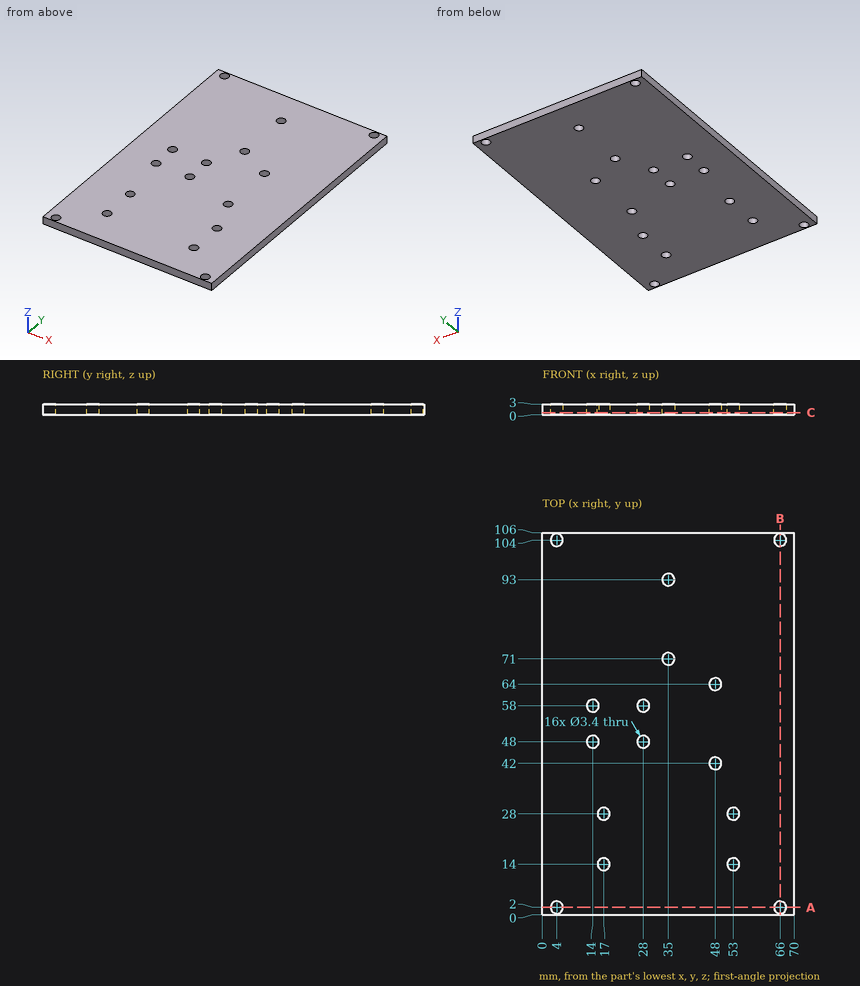
Part print with two shaded views. Sizes in mm from the minimum x, y, z corner. Coordinates: 2 decimals unless noted, no trailing zeros. Write each loop counter-clockwise with the first axis right and the second up, starting at its lowest first coordinate (ties: lowest second). Pieces come first, ordered by that corner, then holes. Notation, with made-up numbers: (-17, 14.25) - (15, 14.25) arc R18 ccw to (15, 48.25) - close; hole circle Ø8 at (16.25, -29.5). An arc over 180 degrees is marked (long way). Put each result on its own line as item: value.
1. Probe line 1 along Y through (x, z) = (66, 1.95); line 2 along Y through (x, z) = (35, 1.7); line 3 along X through (y, z) = (65, 1.7). List the from-to ranges inside material, lowest first. Write a range as [from, to].
Final values:
line 1: y = [0, 0.3], [3.7, 102.3], [105.7, 106]
line 2: y = [0, 69.3], [72.7, 91.3], [94.7, 106]
line 3: x = [0, 46.63], [49.37, 70]
2. Flat gauge pin, fed straight in: pin 1 Ø2 at (x, y) = (53, 28) entering from -Z. Where does the tip first touch, or does it go through?
Final values:
pin 1: passes through
3. Band-saw the part on B-B (x = 66). Write the cut outline in (y, z), then the cut area to 3 significant figures.
Final values:
outline: (0, 0) - (0.3, 0) - (0.3, 3) - (0, 3) - close; (3.7, 0) - (102.3, 0) - (102.3, 3) - (3.7, 3) - close; (105.7, 0) - (106, 0) - (106, 3) - (105.7, 3) - close
area: 298 mm²
4. Band-saw the part on A-A (y = 2). Write the cut outline in (x, z), then the cut area to 3 significant figures.
Final values:
outline: (0, 0) - (2.3, 0) - (2.3, 3) - (0, 3) - close; (5.7, 0) - (64.3, 0) - (64.3, 3) - (5.7, 3) - close; (67.7, 0) - (70, 0) - (70, 3) - (67.7, 3) - close
area: 190 mm²
5. Band-saw the part on C-C (z = 0.6). Give the number of separate pieces and of enclosed holes in the cut face, then the cut area to 3 significant figures.
Final values:
separate pieces: 1
enclosed holes: 16
area: 7,270 mm²
